Geometry: final body of the model. Coordinates: model frame, mm. Face numbers are marked on the shaded views. A direction names the side the tool comes from. Coordinates: 2 decimals unless noted, no trailing zeros. Loops run counter-clockwise (first coordinate to the right, second up) from the corner with the lowest first, then second, coordinate; pieces in that order, holes last. Notation, with made-up numbers: (47.5, 28.5) - (77.5, 28.5) arc R20 ccw to (77.5, 65.5) - close; hole circle Ø3 at (-1.5, 48). An arc over 180 degrees is marked (long way). Answer in a Markdown table with one row per item.
from build123d import *

# Parameters (mm, degrees)
EXTRUDE_1_DEPTH     = 82
SKETCH_4_R          = 1.6
CUT_EXTRUDE_1_DEPTH = 10
FILLET_1_R          = 3
SKETCH_5_R          = 1.6
EXTRUDE_2_DEPTH     = 5
EXTRUDE_START       = -5
SKETCH_6_R          = 1.6
EXTRUDE_3_DEPTH     = 5
SKETCH_7_W          = 5.946088912
SKETCH_7_H          = 0.873329624
CUT_EXTRUDE_2_DEPTH = 115.290435775


with BuildPart() as part:
    # 草图1 → 凸台-拉伸1 (new body)
    with BuildSketch(Plane.XY):
        Polygon((25.726329851, -61.543566927), (30.579717439, -71.951690196), (33.889851195, -71.951690196), (-16.077235621, 35.20307328), (-34.077235621, 35.20307328), (-34.077235621, 32.20307328), (-17.988446404, 32.20307328), align=None)
    extrude(amount=EXTRUDE_1_DEPTH)

    # 草图4 → 切除-拉伸1 (cut)
    with BuildSketch(Plane.XZ.offset(-32.20307328)):
        with Locations(Location((-29.077235621, 67, 0), (0, 0, 270))):
            Circle(SKETCH_4_R)
        with Locations(Location((-29.077235621, 15, 0), (0, 0, 270))):
            Circle(SKETCH_4_R)
    extrude(amount=-CUT_EXTRUDE_1_DEPTH, mode=Mode.SUBTRACT)

    # 圆角1
    fillet_1_edges = [part.edges().sort_by_distance(p)[0] for p in [
        (-17.988446404, 32.20307328, 41),
    ]]
    fillet(fillet_1_edges, radius=FILLET_1_R)

    # 草图5 → 凸台-拉伸2 (add)
    with BuildSketch(Plane(origin=(0, 0, 0), x_dir=(-1, 0, 0), z_dir=(0, 0, -1))):
        with BuildLine():
            Line((-25.579717439, -71.79692672), (-30.507550044, -71.79692672))
            Line((-30.507550044, -71.79692672), (-23.756384483, -57.319005451))
            ThreePointArc((-23.756384483, -57.319005451), (-24.108220381, -60.505712257), (-22.452229611, -63.250996092))
            ThreePointArc((-22.452229611, -63.250996092), (-21.029604517, -68.616859667), (-25.579717439, -71.79692672))
        make_face()
        with Locations((-25.579717439, -66.951690196)):
            Circle(SKETCH_5_R, mode=Mode.SUBTRACT)
    extrude(amount=-EXTRUDE_2_DEPTH)

    # 草图6 → 凸台-拉伸3 (add)
    with BuildSketch(Plane.XY.offset(82).offset(EXTRUDE_START)):
        with BuildLine():
            Line((25.579717439, -71.79692672), (30.507550044, -71.79692672))
            Line((30.507550044, -71.79692672), (23.756384483, -57.319005451))
            ThreePointArc((23.756384483, -57.319005451), (24.108220381, -60.505712257), (22.452229611, -63.250996092))
            ThreePointArc((22.452229611, -63.250996092), (21.029604517, -68.616859667), (25.579717439, -71.79692672))
        make_face()
        with Locations(Location((25.579717439, -66.951690196, 0), (0, 0, 180))):
            Circle(SKETCH_6_R, mode=Mode.SUBTRACT)
    extrude(amount=EXTRUDE_3_DEPTH)

    # 草图7 → 切除-拉伸2 (cut, through all)
    with BuildSketch(Plane.XY.offset(82)):
        with Locations((33.4805945, -72.233591532)):
            Rectangle(SKETCH_7_W, SKETCH_7_H)
    extrude(amount=-CUT_EXTRUDE_2_DEPTH, mode=Mode.SUBTRACT)


solid = part.part
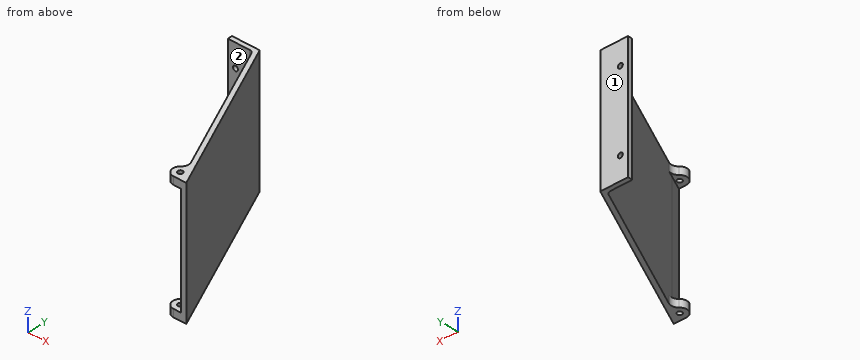
(1) Cut plane B-B on z = 50.5. Output: boundary loops of the cut face in (x, y), then the cut area to 3 significant figures.
Verdict:
| item | result |
|---|---|
| outline | (-34.08, 32.2) - (-19.9, 32.2) arc R3 cw to (-17.18, 30.47) - (30.51, -71.8) - (33.82, -71.8) - (-16.08, 35.2) - (-34.08, 35.2) - close |
| area | 401 mm² |
(2) Cut plane C-C on x = -5.5. Output: boundary loops of the cut face in (y, z), then the cut area to 3 significant figures.
Verdict:
| item | result |
|---|---|
| outline | (5.42, 0) - (12.52, 0) - (12.52, 82) - (5.42, 82) - close |
| area | 582 mm² |
(3) Cut plane D-D on y = -10.5. Output: boundary loops of the cut face in (x, z).
Verdict:
| item | result |
|---|---|
| outline | (1.92, 0) - (5.23, 0) - (5.23, 82) - (1.92, 82) - close |
(4) Access query for the marked faces 1 and 2. Directions: +Z, -Z, +X, -X, +Y, -Y. A direction counts if a zero-diameter tool reaches every point of the face in a straight line with its end or side. Return the directions, or none.
Verdict:
| item | result |
|---|---|
| face 1 | +Z, -Z, +X, -X, +Y |
| face 2 | +Z, -Z, -X, -Y |
(5) Cut plane A-A on z = 15. Output: boundary loops of the cut face in (x, y).
Verdict:
| item | result |
|---|---|
| outline | (-34.08, 32.2) - (-30.68, 32.2) - (-30.68, 35.2) - (-34.08, 35.2) - close; (-27.48, 32.2) - (-19.9, 32.2) arc R3 cw to (-17.18, 30.47) - (30.51, -71.8) - (33.82, -71.8) - (-16.08, 35.2) - (-27.48, 35.2) - close |
(6) Ray query, probe 1 along Y at (x, z) = (-28, 33); probe 2 along Y at (x, z) = (19, 68.5); probe 3 along X at (y, z) = (-48.5, 75). Return the intervals inside material, ascending.
Verdict:
| item | result |
|---|---|
| probe 1 | y = 32.2 to 35.2 |
| probe 2 | y = -47.12 to -40.02 |
| probe 3 | x = 19.64 to 22.95 |
(7) First-contact query: pin 1 Ø3.5 at (x, y) = (25.58, -66.95) entering from -Z; pin 2 Ø4 at (x, z) = (-29.08, 15) entering from -Y; pin 3 Ø5 at (y, z) = (-7.5, 54) entering from +X; pin 4 Ø4 at (x, z) = (23, 10.5) entering from -Y. Flat tips, straight axial feed; report the tip coordinate or a pass-through.
Verdict:
| item | result |
|---|---|
| pin 1 | stops at z = 0 |
| pin 2 | stops at y = 32.2 |
| pin 3 | stops at x = 5 |
| pin 4 | stops at y = -59.99 |
